For this review, take the finished solid that the model builds, in its own axes (mm). A direction names the side the tool comes from. Coordinates: 2 decimals unless noted, no trailing zeros. Loops run counter-clockwise (first coordinate to the right, second up) from the corner with the lowest first, then second, coordinate; pieces in that order, holes last. Notation, with made-up numbers: (-15, 5) - (44, 5) arc R19 ccw to (44, 15) - close; hole circle Ø6 at (0.25, 0.25). An arc over 180 degrees is marked (long way). One line per item, written item: value. Start each with the question number.
1. For faces 1 (the face through (-27, 28, 20)), 2 (the face through (0, 13, 8)), 3 (the face through (-56, 19, 10)), list the 3-axis set-ups (+Z, -Z, +X, -X, +Y, -Y) from which the entire face can be reached by the end or side of a thin tool; tool diameter is ignored.
2. Take a section at A-A, the plane x = -26.75. State the section outline as (y, z) points.
3. To check wall thickness, follow line 1 (Y direction, x = -10, z = 17.25); line 2 (Y direction, x = -26.75, z = 1.3); line 3 (X direction, y = 11.5, z = 13). State the ranges of each line that lie inside material, in increasing order. Write a range as from..to.
4. Insertion check: pin 1 (1.2 mm diameter, centred on x = -56.5, y = 22, fed in from +Z); pin 2 (4.5 mm diameter, centred on x = -55.5, y = 12.5, fed in from +Z). Each pin has a flat end and moves straight along its axis. Give the tip position at first contact, or say it passes through.
5. Take a section at D-D, the plane z = 17.5. State the section outline as (x, y) points.
6. Take a section at C-C, the plane y = 13. State the section outline as (x, z) points.
7. The part is to be moulded in two halves that separate along Y. For faces 4 (the face through (-27, 17, 0)), 5 (the face through (-27, -4, 10)), 6 (the face through (-53.5, 13, 8)), say which applies: released by +Y, released by -Y, zero draft, split by the parting line, or undercut.
8. Take a section at B-B, the plane z = 10. State the section outline as (x, y) points, and give its area (3 significant figures).
```python
from build123d import *

# Parameters (mm, degrees)
SCHIZZO1_W                   = 61.5
SCHIZZO1_H                   = 34
SCHIZZO1_W_2                 = 53.5
SCHIZZO1_H_2                 = 26
ESTRUSIONE_SOTTILE1_DEPTH    = 20
SCHIZZO2_W                   = 53.5
SCHIZZO2_H                   = 26
ESTRUSIONE_ESTRUSIONE1_DEPTH = 4
SCHIZZO3_R                   = 2
TAGLIO_ESTRUSIONE1_DEPTH     = 4
TAGLIO_ESTRUSIONE3_DEPTH     = 72.289901108
SMUSSO1_SIZE                 = 2.2


with BuildPart() as part:
    # Schizzo1 → Estrusione-Sottile1 (new body)
    with BuildSketch(Plane.XY):
        with Locations((-26.75, 13)):
            Rectangle(SCHIZZO1_W, SCHIZZO1_H)
        with Locations((-26.75, 13)):
            Rectangle(SCHIZZO1_W_2, SCHIZZO1_H_2, mode=Mode.SUBTRACT)
    extrude(amount=ESTRUSIONE_SOTTILE1_DEPTH)

    # Schizzo2 → Estrusione-Estrusione1 (add)
    with BuildSketch(Plane.XY):
        with Locations((-26.75, 13)):
            Rectangle(SCHIZZO2_W, SCHIZZO2_H)
    extrude(amount=ESTRUSIONE_ESTRUSIONE1_DEPTH)

    # Schizzo3 → Taglio-Estrusione1 (cut)
    with BuildSketch(Plane.XY.offset(4)):
        with Locations((-26.75, 13)):
            Circle(SCHIZZO3_R)
    extrude(amount=-TAGLIO_ESTRUSIONE1_DEPTH, mode=Mode.SUBTRACT)

    # Schizzo4 → Taglio-Estrusione3 (cut, through all)
    with BuildSketch(Plane.ZY.offset(57.5)):
        Polygon((20, 110.783466983), (20, 27), (20, 25), (6.250230313, 25), (6.250230313, 19), (14.445683016, 19), (14.445683016, 7), (6.250230313, 7), (6.250230313, 1), (20, 1), (20, -1), (20, -84.783466983), (187.566933966, -84.783466983), (187.566933966, 110.783466983), align=None)
    extrude(amount=-TAGLIO_ESTRUSIONE3_DEPTH, mode=Mode.SUBTRACT)

    # Smusso1
    smusso1_edges = [part.edges().sort_by_distance(p)[0] for p in [
        (-28.75, 13, 4),
    ]]
    chamfer(smusso1_edges, length=SMUSSO1_SIZE)


solid = part.part
```
Solutions:
1. face 1: +Z, +X, -X, +Y, -Y
1. face 2: +Z
1. face 3: +Z, +X, -X
2. outline: (-4, 0) - (11, 0) - (11, 1.8) - (8.8, 4) - (0, 4) - (0, 20) - (-4, 20) - close; (15, 0) - (30, 0) - (30, 20) - (26, 20) - (26, 4) - (17.2, 4) - (15, 1.8) - close
3. line 1: -4..0, 26..30
3. line 2: -4..11, 15..30
3. line 3: -57.5..-53.5, 0..4
4. pin 1: z = 6.25
4. pin 2: z = 14.45
5. outline: (-57.5, -4) - (4, -4) - (4, 1) - (0, 1) - (0, 0) - (-53.5, 0) - (-53.5, 1) - (-57.5, 1) - close; (-57.5, 25) - (-53.5, 25) - (-53.5, 26) - (0, 26) - (0, 25) - (4, 25) - (4, 30) - (-57.5, 30) - close
6. outline: (-57.5, 0) - (-28.75, 0) - (-28.75, 1.8) - (-30.95, 4) - (-53.5, 4) - (-53.5, 14.45) - (-57.5, 14.45) - close; (-24.75, 0) - (4, 0) - (4, 14.45) - (0, 14.45) - (0, 4) - (-22.55, 4) - (-24.75, 1.8) - close
7. face 4: zero draft
7. face 5: released by -Y
7. face 6: undercut
8. outline: (-57.5, -4) - (4, -4) - (4, 1) - (0, 1) - (0, 0) - (-53.5, 0) - (-53.5, 1) - (-57.5, 1) - close; (-57.5, 7) - (-53.5, 7) - (-53.5, 19) - (-57.5, 19) - close; (-57.5, 25) - (-53.5, 25) - (-53.5, 26) - (0, 26) - (0, 25) - (4, 25) - (4, 30) - (-57.5, 30) - close; (0, 7) - (4, 7) - (4, 19) - (0, 19) - close
8. area: 604 mm2
